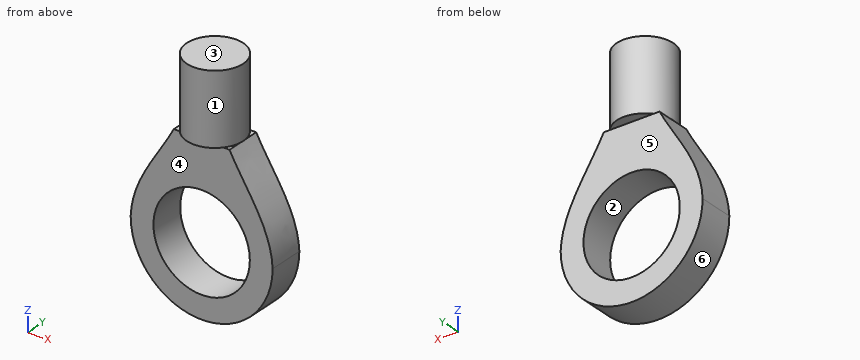
from build123d import *

# Parameters (mm, degrees)
SKETCH2_R           = 8.15
BOSS_EXTRUDE1_DEPTH = 6
SKETCH3_R           = 4.755
BOSS_EXTRUDE2_DEPTH = 12


with BuildPart() as part:
    # Sketch2 → Boss-Extrude1 (new body)
    with BuildSketch(Plane(origin=(0, 0, 0), x_dir=(1, 0, 0), z_dir=(0, 1, 0))):
        with BuildLine():
            Line((-4.71, -15.99), (4.71, -15.99))
            add(Edge.make_bspline(
                [(12, 0), (11.768004517, -6.147027332), (7.327289648, -10.952825214), (4.71, -15.99)],
                knots=[0, 0, 0, 0, 0.424868327, 0.424868327, 0.424868327, 0.424868327], degree=3))
            ThreePointArc((12, 0), (0, 12), (-12, 0))
            add(Edge.make_bspline(
                [(-12, 0), (-11.768004517, -6.147027332), (-7.327289648, -10.952825214), (-4.71, -15.99)],
                knots=[0, 0, 0, 0, 0.424868327, 0.424868327, 0.424868327, 0.424868327], degree=3))
        make_face()
        Circle(SKETCH2_R, mode=Mode.SUBTRACT)
    extrude(amount=BOSS_EXTRUDE1_DEPTH)

    # Sketch3 → Boss-Extrude2 (add)
    with BuildSketch(Plane.XY.offset(15.99)):
        with Locations((0, 3)):
            Circle(SKETCH3_R)
    extrude(amount=BOSS_EXTRUDE2_DEPTH)


solid = part.part
The model under review builds one solid part; all positions refer to its coordinate system, in mm. Face numbers are marked on the shaded views. A direction names the side the tool comes from. Coordinates: 2 decimals unless noted, no trailing zeros. Write each loop counter-clockwise with the first axis right and the second up, starting at its lowest first coordinate (ties: lowest second). Pieces come first, ordered by that corner, then holes. Notation, with made-up numbers: (54.25, 2) - (104.25, 2) arc R21 ccw to (104.25, 39) - close; hole circle Ø5 at (-33, 34). An arc over 180 degrees is marked (long way). Answer as a JSON object with one key per item and string values. Group by question number.
1. Clearance check with flat-ended pins moving along their axes: pin 1 Ø2 at (x, y) = (-9, 5) entering from -Z; pin 2 Ø1.9 at (x, y) = (1.5, -1) entering from -Z; pin 3 Ø2 at (x, y) = (6.5, 4) entering from +Z. State where each tip first meets the part, or that it passes through.
2. Add section A-A (x = 0). Give the boundary of the cut face in (y, z) (3 decimals), plus the area to 3 significant figures.
3. Machinability: for the marked faces 4, 5 and 6, which of the approach directions +Z, -Z, +X, -X, +Y, -Y give a long, thin tool a straight path to every point of the face, cutting with its end or side? Answer none if there is none.
4. Add section B-B (z = -5). Give the boundary of the cut face in (x, y), plus the area to 3 significant figures.
5. To check wall thickness, follow probe 1 along Z at (x, y) = (0, 3.85); probe 2 along X at (y, z) = (3.25, 25.5); probe 3 along X at (y, z) = (4.75, -3). State the ranges of each line that lie inside material, in increasing order.
6. Mouldability with a two-part tool opening along X and no side actions: class the marked faces 1, 2 and 3 as pulls with the +X half, pulls with the -X half, needs draft (parallel to the pull), parting line crosses it, or undercut.
7. Add section D-D (y = 7). Give the boundary of the cut face in (x, z), plus the area to 3 significant figures.
8. Add section C-C (z = -0.5). Give the boundary of the cut face in (x, y).
Findings:
{
 "1": {"pin 1": "z = -8.94", "pin 2": "z = 15.99", "pin 3": "z = 14.56"},
 "2": {"outline": "(-1.755, 15.99) - (0, 15.99) - (0, 8.15) - (6, 8.15) - (6, 15.99) - (7.755, 15.99) - (7.755, 27.99) - (-1.755, 27.99) - close; (0, -12) - (6, -12) - (6, -8.15) - (0, -8.15) - close", "area": "184 mm²"},
 "3": {"face 4": "-Z, +X, -X, -Y", "face 5": "-Z, +X, -X, +Y", "face 6": "-Z, +Y, -Y"},
 "4": {"outline": "(-10.91, 0) - (-6.44, 0) - (-6.44, 6) - (-10.91, 6) - close; (6.44, 0) - (10.91, 0) - (10.91, 6) - (6.44, 6) - close", "area": "53.7 mm²"},
 "5": {"probe 1": "-12 to -8.15, 8.15 to 27.99", "probe 2": "-4.75 to 4.75", "probe 3": "-11.62 to -7.58, 7.58 to 11.62"},
 "6": {"face 1": "parting line crosses it", "face 2": "undercut", "face 3": "needs draft"},
 "7": {"outline": "(-2.57, 15.99) - (2.57, 15.99) - (2.57, 27.99) - (-2.57, 27.99) - close", "area": "61.7 mm²"},
 "8": {"outline": "(-11.99, 0) - (-8.13, 0) - (-8.13, 6) - (-11.99, 6) - close; (8.13, 0) - (11.99, 0) - (11.99, 6) - (8.13, 6) - close"}
}
